The listing builds one solid part. Answer for the finished solid, in the listing's coordinates (mm). A direction names the side the tool comes from. Give positions to 0.01 mm unless a question says otherwise; leave off trailing zeros. Write each loop counter-clockwise with the first axis right and the second up, starting at its lowest first coordinate (ties: lowest second). Pieces come first, ordered by that corner, then holes. Notation, with made-up numbers: (-36, 22) - (-1, 22) arc R32 cw to (-1, 53) - close; hole circle Ø6 at (-17.75, 52). An arc over 180 degrees is marked (long way). Use a Markdown table: item, result. Add a question column.
from build123d import *

# Parameters (mm, degrees)
SKETCH1_W           = 40
SKETCH1_H           = 40
BOSS_EXTRUDE1_DEPTH = 3
CUT_EXTRUDE1_DEPTH  = 1.5
SKETCH3_R           = 2.5
CUT_EXTRUDE2_DEPTH  = 2.5
FILLET1_R           = 5
SKETCH4_W           = 40
SKETCH4_H           = 8
CUT_EXTRUDE3_DEPTH  = 2


with BuildPart() as part:
    # Sketch1 → Boss-Extrude1 (new body)
    with BuildSketch(Plane(origin=(0, 0, 0), x_dir=(1, 0, 0), z_dir=(0, 1, 0))):
        Rectangle(SKETCH1_W, SKETCH1_H)
    extrude(amount=BOSS_EXTRUDE1_DEPTH)

    # Sketch2 → Cut-Extrude1 (cut)
    with BuildSketch(Plane(origin=(0, 3, 0), x_dir=(1, 0, 0), z_dir=(0, 1, 0))):
        with BuildLine():
            ThreePointArc((-5, 10), (-13.535533906, 13.535533906), (-10, 5))
            Line((-10, 5), (-10, 10))
            Line((-10, 10), (-5, 10))
        make_face()
        with BuildLine():
            Line((-10, 10), (-10, 5))
            ThreePointArc((-10, 5), (-6.464466094, 6.464466094), (-5, 10))
            Line((-5, 10), (-10, 10))
        make_face()
        with BuildLine():
            ThreePointArc((5, 10), (6.464466094, 6.464466094), (10, 5))
            Line((10, 5), (10, 10))
            Line((10, 10), (5, 10))
        make_face()
        with BuildLine():
            Line((10, 10), (10, 5))
            ThreePointArc((10, 5), (13.535533906, 6.464466094), (15, 10))
            ThreePointArc((15, 10), (10, 15), (5, 10))
            Line((5, 10), (10, 10))
        make_face()
        with BuildLine():
            Line((-10, -5), (-10, -10))
            Line((-10, -10), (-5, -10))
            ThreePointArc((-5, -10), (-6.464466094, -6.464466094), (-10, -5))
        make_face()
        with BuildLine():
            Line((-5, -10), (-10, -10))
            Line((-10, -10), (-10, -5))
            ThreePointArc((-10, -5), (-13.535533906, -13.535533906), (-5, -10))
        make_face()
        with BuildLine():
            ThreePointArc((10, -5), (6.464466094, -6.464466094), (5, -10))
            Line((5, -10), (10, -10))
            Line((10, -10), (10, -5))
        make_face()
        with BuildLine():
            Line((10, -10), (5, -10))
            ThreePointArc((5, -10), (10, -15), (15, -10))
            ThreePointArc((15, -10), (13.535533906, -6.464466094), (10, -5))
            Line((10, -5), (10, -10))
        make_face()
    extrude(amount=-CUT_EXTRUDE1_DEPTH, mode=Mode.SUBTRACT)

    # Sketch3 → Cut-Extrude2 (cut, through all)
    with BuildSketch(Plane(origin=(0, 1.5, 0), x_dir=(1, 0, 0), z_dir=(0, 1, 0))):
        with Locations((-10, 10)):
            Circle(SKETCH3_R)
        with Locations((10, 10)):
            Circle(SKETCH3_R)
        with Locations((-10, -10)):
            Circle(SKETCH3_R)
        with Locations((10, -10)):
            Circle(SKETCH3_R)
    extrude(amount=-CUT_EXTRUDE2_DEPTH, mode=Mode.SUBTRACT)

    # Fillet1
    fillet1_edges = [part.edges().sort_by_distance(p)[0] for p in [
        (20, 1.5, 20),
        (-20, 1.5, 20),
        (-20, 1.5, -20),
        (20, 1.5, -20),
    ]]
    fillet(fillet1_edges, radius=FILLET1_R)

    # Sketch4 → Cut-Extrude3 (cut)
    with BuildSketch(Plane(origin=(0, 3, 0), x_dir=(1, 0, 0), z_dir=(0, 1, 0))):
        Rectangle(SKETCH4_W, SKETCH4_H)
    extrude(amount=-CUT_EXTRUDE3_DEPTH, mode=Mode.SUBTRACT)


solid = part.part
1. The part is cut by section A-A (y = 2.35). Give the vertices of the cut face in (x, z).
2. Given P1, Ø6, axis at x = -11, z = -2, coming from the -Y side; P2, Ø3, axis at x = -11.5, z = 9.5, coming from the +Y side, each flat-ended and moving along its own axis, determine where each tip first touches the part or whether it passes through.
3. Consider L1, parallel to Z at x = -10, y = 2.4; L2, parallel to X at y = 0.45, z = 10; L3, parallel to Z at x = -10, y = 1.05. Determine where each line is inside the solid, lowest interval first. Write a range as [from, to].
4. Which of the six approach directions +Z, -Z, +X, -X, +Y, -Y give full straight-line access (tool end or side, diameter ignored) to faces 4 (the flat face through (-8, 1.5, 12)), 5 (the flat face through (0, 2, 4)), 6 (the flat face through (0, 0, 0))?
5. For a pull along X with two mould halves and no side action, classify faces 1 (the flat face through (-8, 1.5, -8)), 2 (the flat face through (0, 3, -12)), 3 (the cylindrical face through (18, 2, 19)) as released by +X, released by -X, zero draft, split by the parting line, or undercut.
6. The part is cut by section D-D (x = 8). Give the vertices of the cut face in (y, z).
7. The part is cut by section B-B (x = 3). Give the vertices of the cut face in (y, z), and give its area (3 significant figures).
8. The part is cut by section C-C (z = 9.5). Give the vertices of the cut face in (x, y).
Check values:
| question | item | result |
|---|---|---|
| 1 | outline | (-20, -15) arc R5 ccw to (-15, -20) - (15, -20) arc R5 ccw to (20, -15) - (20, -4) - (-20, -4) - close; (-20, 4) - (20, 4) - (20, 15) arc R5 ccw to (15, 20) - (-15, 20) arc R5 ccw to (-20, 15) - close; hole circle Ø10 at (-10, -10); hole circle Ø10 at (-10, 10); hole circle Ø10 at (10, -10); hole circle Ø10 at (10, 10) |
| 2 | P1 | stops at y = 0 |
| 2 | P2 | stops at y = 1.5 |
| 3 | L1 | z = [-20, -15], [-5, -4], [4, 5], [15, 20] |
| 3 | L2 | x = [-20, -12.5], [-7.5, 7.5], [12.5, 20] |
| 3 | L3 | z = [-20, -12.5], [-7.5, -4], [4, 7.5], [12.5, 20] |
| 4 | face 4 | +Y |
| 4 | face 5 | +X, -X, +Y |
| 4 | face 6 | +Z, -Z, +X, -X, -Y |
| 5 | face 1 | undercut |
| 5 | face 2 | zero draft |
| 5 | face 3 | released by +X |
| 6 | outline | (0, -20) - (3, -20) - (3, -14.58) - (1.5, -14.58) - (1.5, -11.5) - (0, -11.5) - close; (0, -8.5) - (1.5, -8.5) - (1.5, -5.42) - (3, -5.42) - (3, -4) - (1, -4) - (1, 4) - (3, 4) - (3, 5.42) - (1.5, 5.42) - (1.5, 8.5) - (0, 8.5) - close; (0, 11.5) - (1.5, 11.5) - (1.5, 14.58) - (3, 14.58) - (3, 20) - (0, 20) - close |
| 7 | outline | (0, -20) - (3, -20) - (3, -4) - (1, -4) - (1, 4) - (3, 4) - (3, 20) - (0, 20) - close |
| 7 | area | 104 mm2 |
| 8 | outline | (-20, 0) - (-12.45, 0) - (-12.45, 1.5) - (-14.97, 1.5) - (-14.97, 3) - (-20, 3) - close; (-7.55, 0) - (7.55, 0) - (7.55, 1.5) - (5.03, 1.5) - (5.03, 3) - (-5.03, 3) - (-5.03, 1.5) - (-7.55, 1.5) - close; (12.45, 0) - (20, 0) - (20, 3) - (14.97, 3) - (14.97, 1.5) - (12.45, 1.5) - close |
